```python
from build123d import *

# Parameters (mm, degrees)
FILLET_1_R          = 2
CHAMFER_1_SIZE      = 2
CUT_EXTRUDE_1_DEPTH = 43
CUT_EXTRUDE_2_DEPTH = 47


with BuildPart() as part:
    # 草图1 → 旋转1 (revolve)
    with BuildSketch(Plane(origin=(0, 0, 0), x_dir=(0, 0, -1), z_dir=(1, 0, 0)), mode=Mode.PRIVATE) as revolve_1_sk:
        with BuildLine():
            Line((-165, 0), (-165, -22.5))
            Line((-165, -22.5), (-120, -22.5))
            Line((-120, -22.5), (-120, -23.5))
            Line((-120, -23.5), (0, -23.5))
            Line((0, -23.5), (0, -26))
            Line((0, -26), (90, -26))
            Line((90, -26), (90, -23))
            ThreePointArc((90, -23), (90.234314575, -22.434314575), (90.8, -22.2))
            Line((90.8, -22.2), (91.7, -22.2))
            Line((91.7, -22.2), (92, -22.5))
            Line((92, -22.5), (133, -22.5))
            Line((133, -22.5), (133, -21.5))
            Line((133, -21.5), (183, -21.5))
            Line((183, -21.5), (183, -21))
            Line((183, -21), (293, -21))
            Line((293, -21), (293, 0))
            Line((293, 0), (-165, 0))
        make_face()
    revolve(revolve_1_sk.sketch.rotate(Axis((0, 0, 440.995541918), (0, 0, -1)), 270), axis=Axis((0, 0, 440.995541918), (0, 0, -1)))

    # 圆角1
    # the kernel refuses this fillet: 2 mm, written as the material it adds along each edge
    with BuildSketch(Plane(origin=(0, 0, 120), x_dir=(1, 0, 0), z_dir=(0, 1, 0))) as fillet_1_piece_1:
        with BuildLine():
            CenterArc((24.5, -1.732050808), FILLET_1_R, 120, 60)
            Line((23.5, 0), (23.48, 0.034641016))
            ThreePointArc((23.48, 0.034641016), (23, 0.04), (22.5, 0.04))
            Line((22.5, 0.04), (22.46, 0))
            Line((22.46, 0), (22.46, -1.732050808))
            Line((22.46, -1.732050808), (22.5, -1.732050808))
        make_face()
    revolve(axis=Axis((0, 0, 120), (0, 0, -1)))
    with BuildSketch(Plane(origin=(0, 0, 0), x_dir=(1, 0, 0), z_dir=(0, 1, 0))) as fillet_1_piece_2:
        with BuildLine():
            CenterArc((23.5 + FILLET_1_R, -FILLET_1_R), FILLET_1_R, 90, 90)
            Line((23.5 + FILLET_1_R, 0), (23.5 + FILLET_1_R, FILLET_1_R * 0.02))
            Line((23.5 + FILLET_1_R, FILLET_1_R * 0.02), (23.5 - FILLET_1_R * 0.02, FILLET_1_R * 0.02))
            Line((23.5 - FILLET_1_R * 0.02, FILLET_1_R * 0.02), (23.5 - FILLET_1_R * 0.02, -FILLET_1_R))
            Line((23.5 - FILLET_1_R * 0.02, -FILLET_1_R), (23.5, -FILLET_1_R))
        make_face()
    revolve(axis=Axis((0, 0, 0), (0, 0, -1)))
    with BuildSketch(Plane(origin=(0, 0, -133), x_dir=(1, 0, 0), z_dir=(0, 1, 0))) as fillet_1_piece_3:
        with BuildLine():
            CenterArc((23.5, 1.732050808), FILLET_1_R, 180, 60)
            Line((21.5, 1.732050808), (21.46, 1.732050808))
            Line((21.46, 1.732050808), (21.46, 0))
            Line((21.46, 0), (21.5, -0.04))
            ThreePointArc((21.5, -0.04), (22, -0.04), (22.48, -0.034641016))
            Line((22.48, -0.034641016), (22.5, 0))
        make_face()
    revolve(axis=Axis((0, 0, -133), (0, 0, -1)))
    with BuildSketch(Plane(origin=(0, 0, -183), x_dir=(1, 0, 0), z_dir=(0, 1, 0))) as fillet_1_piece_4:
        with BuildLine():
            CenterArc((23, 1.322875656), FILLET_1_R, 180, 41.409622109)
            Line((21, 1.322875656), (20.96, 1.322875656))
            Line((20.96, 1.322875656), (20.96, 0))
            Line((20.96, 0), (21, -0.04))
            ThreePointArc((21, -0.04), (21.25, -0.04), (21.47, -0.026457513))
            Line((21.47, -0.026457513), (21.5, 0))
        make_face()
    revolve(axis=Axis((0, 0, -183), (0, 0, -1)))

    # 倒角1
    chamfer_1_edges = [part.edges().sort_by_distance(p)[0] for p in [
        (-22.5, 0, 165),
        (-21, 0, -293),
    ]]
    chamfer(chamfer_1_edges, length=CHAMFER_1_SIZE)

    # 草图3 → 切除-拉伸1 (cut)
    with BuildSketch(Plane(origin=(18, 0, 0), x_dir=(0, 0, -1), z_dir=(1, 0, 0))):
        with BuildLine():
            Line((-109, 7), (-13, 7))
            ThreePointArc((-13, 7), (-6, 0), (-13, -7))
            Line((-13, -7), (-109, -7))
            ThreePointArc((-109, -7), (-116, 0), (-109, 7))
        make_face()
    extrude(amount=CUT_EXTRUDE_1_DEPTH, mode=Mode.SUBTRACT)

    # 草图4 → 切除-拉伸2 (cut)
    with BuildSketch(Plane(origin=(16, 0, 0), x_dir=(0, 0, -1), z_dir=(1, 0, 0))):
        with BuildLine():
            Line((199, 6), (293, 6))
            Line((293, 6), (293, -6))
            Line((293, -6), (199, -6))
            ThreePointArc((199, -6), (193, 0), (199, 6))
        make_face()
    extrude(amount=CUT_EXTRUDE_2_DEPTH, mode=Mode.SUBTRACT)


solid = part.part
```
The listing builds one solid part. Answer for the finished solid, in the listing's coordinates (mm). A direction names the side the tool comes from. Coordinates: 2 decimals unless noted, no trailing zeros. Loops run counter-clockwise (first coordinate to the right, second up) from the corner with the lowest first, then second, coordinate; pieces in that order, holes last. Notation, with made-up numbers: (67.25, 10.25) -> (115.25, 10.25) arc R13 ccw to (115.25, 21.25) -> close; hole circle Ø1 at (17, 32). An arc over 180 degrees is marked (long way). Return JSON: item names as keys, results as strings. Group by question number.
(1) Determine the mould class of faces 6 (the flat face through (18, 0, 60)), 7 (the cylindrical face through (-17.32, -15.88, 60.17)), 8 (the flat face through (0, 0, 165)) for opening direction Y: released by +Y, released by -Y, zero draft, split by the parting line, or undercut.
(2) Which of the six approach directions +Z, -Z, +X, -X, +Y, -Y give full straight-line access (tool end or side, diameter ignored) to faces 1 (the flat face through (16, 0, -244)), 2 (the cylindrical face through (21, 0, 6)), 3 (the cylindrical face through (20.784, 8.618, 142.077)), 4 (the cylindrical face through (11.93, -18.72, -91.26)), 5 (the cylindrical face through (20.784, 8.618, -112.787))?
(3) Given pin 1 Ø3.5 at (y, z) = (-3, -235) entering from +X; pin 2 Ø2 at (x, z) = (19, -250.5) entering from +Y; pin 3 Ø2 at (x, y) = (19.5, -15.5) entering from +Z, each flat-ended and moving along its own axis, determine where each tip first touches the part or whether it passes through.
(4) A cutting plane is placed at A-A on z = -162. Write down the section's boundary in (x, y).
(5) A cutting plane is placed at B-B on z = 21. Write down the section's boundary in (x, y), and give its area (3 significant figures).
(6) Find the intervals of material crossed by probe 1 along X at (y, z) = (1.5, 82); probe 2 along X at (y, z) = (16, -43.5); probe 3 along Y at (x, z) = (11, -48), in increasing order. Write a range as from..to.
The answers:
{
 "1": {"face 6": "undercut", "face 7": "split by the parting line", "face 8": "zero draft"},
 "2": {"face 1": "-Z, +X", "face 2": "+X", "face 3": "+Z", "face 4": "none", "face 5": "-Z"},
 "3": {"pin 1": "stops at x = 16", "pin 2": "stops at y = 10.82", "pin 3": "stops at z = 0.79"},
 "4": {"outline": "circle Ø43 at (0, 0)"},
 "5": {"outline": "(18, -7) -> (18, 7) -> (22.43, 7) arc R23.5 ccw (long way) to (22.43, -7) -> close", "area": "1,660 mm^2"},
 "6": {"probe 1": "x = -23.45..18", "probe 2": "x = -20.49..20.49", "probe 3": "y = -23.56..23.56"}
}
